```python
from build123d import *

# Parameters (mm, degrees)
SKETCH1_W               = 620
SKETCH1_H               = 820
SKETCH1_W_2             = 600
SKETCH1_H_2             = 800
EXTRUDE_THIN1_DEPTH     = 450
SKETCH2_W               = 610
SKETCH2_H               = 5
CUT_EXTRUDE1_DEPTH      = 1000
CUT_EXTRUDE1_DEPTH_BACK = 1000
SKETCH3_R               = 10
CUT_EXTRUDE2_DEPTH      = 3


with BuildPart() as part:
    # Sketch1 → Extrude-Thin1 (new body)
    with BuildSketch(Plane.XY):
        with Locations((300, 400)):
            Rectangle(SKETCH1_W, SKETCH1_H)
        with Locations((300, 400)):
            Rectangle(SKETCH1_W_2, SKETCH1_H_2, mode=Mode.SUBTRACT)
    extrude(amount=EXTRUDE_THIN1_DEPTH)

    # Sketch2 → Cut-Extrude1 (cut, two sides)
    with BuildSketch(Plane.XY) as cut_extrude1_sk:
        with Locations((300, 602.200684115)):
            Rectangle(SKETCH2_W, SKETCH2_H)
        with Locations((300, 792.200684115)):
            Rectangle(SKETCH2_W, SKETCH2_H)
        with Locations((300, 412.200684115)):
            Rectangle(SKETCH2_W, SKETCH2_H)
        with Locations((300, 222.200684115)):
            Rectangle(SKETCH2_W, SKETCH2_H)
    extrude(amount=CUT_EXTRUDE1_DEPTH, mode=Mode.SUBTRACT)
    extrude(cut_extrude1_sk.sketch, amount=-CUT_EXTRUDE1_DEPTH_BACK, mode=Mode.SUBTRACT)

    # Sketch3 → Cut-Extrude2 (cut)
    with BuildSketch(Plane(origin=(0, -10, 0), x_dir=(-1, 0, 0), z_dir=(0, -1, 0))):
        with Locations((-560, -50)):
            Circle(SKETCH3_R)
        with Locations((-40, -50)):
            Circle(SKETCH3_R)
        with Locations((-560, -400)):
            Circle(SKETCH3_R)
        with Locations((-40, -400)):
            Circle(SKETCH3_R)
    extrude(amount=-CUT_EXTRUDE2_DEPTH, mode=Mode.SUBTRACT)


solid = part.part
```
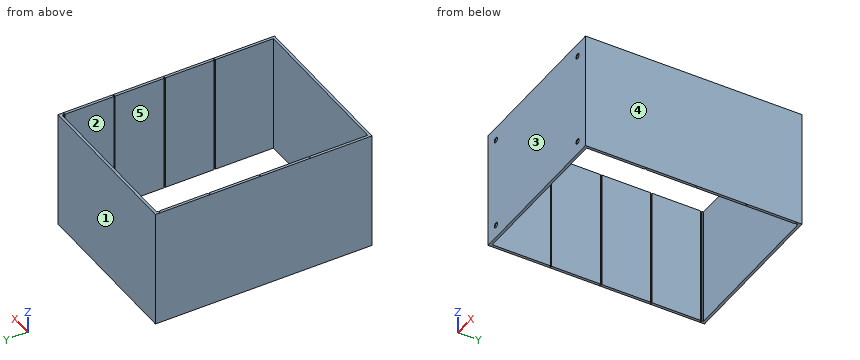
Check sheet for the modelled part. Datum: model origin and axes. Units: mm. Face numbers are marked on the shaded views. A direction names the side the tool comes from. Round coordinates to 2 decimals unless told otherwise and drop trailing zeros. Order: outer loops, then holes, each group sorted by start corner. A loop starts at its lowest first (then second) coordinate and runs counter-clockwise, first axis right, second up.
1) Go/stop test with a flat-tipped pin: pin 1 Ø16 at (x, z) = (560, 50) entering from -Y. Record where the tip stops, or that it passes through.
2) Section check B-B (x = 40). Record the boundary of the cut face in (y, z).
3) Tool access check on the marked faces 1 and 2. Record the directions out of +Z, -Z, +X, -X, +Y, -Y that give a thin tool (end or side, any length) a straight path to the whole face; none if there is none.
4) Scan lines: line 1 (X direction, y = -8.05, z = 50); line 2 (Z direction, x = 40, y = -8.45); line 3 (Y direction, x = 90, z = 423.5). Record each from-to range of solid material in increasing order.
5) Section check C-C (x = 355). Record the boundary of the cut face in (y, z).
6) Mould release check, pull along X, two halves, no side actions. Record for the marked faces 3, 4 and 5: +X half, -X half, draft (parallel to the pull), parting line (faces both ways), or undercut.
7) Section check A-A (y = 368.5). Record the boundary of the cut face in (x, z).
Result:
1. pin 1: stops at y = -7
2. outline: (-10, 0) - (0, 0) - (0, 450) - (-10, 450) - (-10, 410) - (-7, 410) - (-7, 390) - (-10, 390) - (-10, 60) - (-7, 60) - (-7, 40) - (-10, 40) - close; (800, 0) - (810, 0) - (810, 450) - (800, 450) - close
3. face 1: +Z, -Z, +X, -X, +Y
3. face 2: +Z, -Z
4. line 1: x = -10 to 30, 50 to 550, 570 to 610
4. line 2: z = 0 to 40, 60 to 390, 410 to 450
4. line 3: y = -10 to 0, 800 to 810
5. outline: (-10, 0) - (0, 0) - (0, 450) - (-10, 450) - close; (800, 0) - (810, 0) - (810, 450) - (800, 450) - close
6. face 3: draft
6. face 4: +X half
6. face 5: undercut
7. outline: (-10, 0) - (0, 0) - (0, 450) - (-10, 450) - close; (600, 0) - (610, 0) - (610, 450) - (600, 450) - close
